from build123d import *

# Parameters (mm, degrees)
F1_DEPTH = 5
F2_W     = 240
F2_H     = 5
F3_DEPTH = 145
F5_DEPTH = 10
F6_DEPTH = 10


with BuildPart() as f1:
    # F0 (on Top) → F1 (new body)
    with BuildSketch(Plane.XY):
        Polygon((-126.897684, 95.248217), (-131.897684, 95.248217), (-131.897684, -154.751783), (118.102316, -154.751783), (118.102316, 95.248217), (113.102316, 95.248217), (113.102316, 81.383812), (-126.897684, 81.383812), align=None)
    extrude(amount=F1_DEPTH)

    # F2 (on face) → F3 (join)
    with BuildSketch(Plane.XY.offset(5)):
        Polygon((-126.897684, -149.751783), (-126.897684, 95.248217), (-131.897684, 95.248217), (-131.897684, -154.751783), (-126.897684, -154.751783), align=None)
        with Locations((-6.897684, -152.251783)):
            Rectangle(F2_W, F2_H)
        Polygon((113.102316, 95.248217), (113.102316, -149.751783), (113.102316, -154.751783), (118.102316, -154.751783), (118.102316, 95.248217), align=None)
    extrude(amount=F3_DEPTH)

    # F4 (on face) → F5 (join)
    with BuildSketch(Plane.XY.offset(150)):
        Polygon((-128.897684, -151.751783), (-6.897684, -151.751783), (-6.897684, -149.751783), (-126.897684, -149.751783), align=None)
        Polygon((-128.897684, 95.248217), (-128.897684, -151.751783), (-126.897684, -149.751783), (-126.897684, 95.248217), align=None)
    extrude(amount=F5_DEPTH)

    # F4 (on face) → F6 (join)
    with BuildSketch(Plane.XY.offset(150)):
        Polygon((118.102316, 95.248217), (116.102316, 95.248217), (116.102316, -152.751783), (118.102316, -154.751783), align=None)
        Polygon((118.102316, -154.751783), (116.102316, -152.751783), (-6.897684, -152.751783), (-6.897684, -154.751783), align=None)
    extrude(amount=F6_DEPTH)


solid = f1.part
Can you work these out from the model? Positions are in its coordinate system, mm. A direction names the side the tool comes from. Give positions to 0.01 mm unless a question says otherwise; leave off trailing zeros. Loops run counter-clockwise (first coordinate to the right, second up) from the corner with the lowest first, then second, coordinate; pieces in that order, holes last. Notation, with made-up numbers: M 4.5,58.5 L 55.5,58.5 A24 cw 55.5,83.5 Z; hole C -30.75,22 d10. An arc over 180 degrees is marked long. One line per item, written item: value. Start each with the question number.
1) Thinking about a two-plate mould opening in X: for faces 1 (the face through (-128.898, -27, 155)), 2 (the face through (113.102, -26, 74)), 3 (the face through (-9, -154.752, 79)), which applies, +X half, -X half, draft (parallel to the pull), parting line (faces both ways), or undercut?
2) If I drill on line 1 (X direction, y = 28.5, z = 110.5); line 2 (Y direction, x = 70, z = 109.5); line 3 (Z direction, x = -115, y = -28), over which ranges is the centre line in solid material (lowest first)? Write a range as [from, to].
3) I'm going to push flat-ended pins straight in: pin 1 (5.5 mm diameter, centred on x = -44.5, z = 1.5, fed in from +Y); pin 2 (11 mm diameter, centred on x = 49, z = 153.5, fed in from +Y); pin 3 (8 mm diameter, centred on y = -85.5, z = 154.5, fed in from -X); pin 4 (5 mm diameter, centred on x = 83, y = -89, fed in from -Z). Where does each tip first touch, or does it pass through?
4) If we section it at A-A, the plane z = 20: Write out the boundary of the cut face in (x, y), and give its area (3 significant figures).
5) If we section it at B-B, the plane y = -106.5: Write out the boundary of the cut face in (x, z), and give its area (3 significant figures).
6) If we section it at C-C, the plane x = -78.5: Write out the boundary of the cut face in (y, z), and give its area (3 significant figures).
7) On a 3-axis mill with a long thin cutter (end or side, diameter ignored), from which of +Z, -Z, +X, -X, +Y, -Y can I reach the whole of each face in a straight line? I mean faces 4 (the face through (118.102, -32, 79)), 5 (the face through (-69, -151.752, 155)), 6 (the face through (55, -152.752, 155)), 7 (the face through (-9, -33, 5)), 8 (the face through (-131.898, -28, 74)). Say none if no direction works.
Completed:
1. face 1: -X half
1. face 2: undercut
1. face 3: draft
2. line 1: x = [-131.9, -126.9], [113.1, 118.1]
2. line 2: y = [-154.75, -149.75]
2. line 3: z = [0, 5]
3. pin 1: stops at y = 81.38
3. pin 2: stops at y = -149.75
3. pin 3: stops at x = -128.9
3. pin 4: stops at z = 0
4. outline: M -131.9,-154.75 L 118.1,-154.75 L 118.1,95.25 L 113.1,95.25 L 113.1,-149.75 L -126.9,-149.75 L -126.9,95.25 L -131.9,95.25 Z
4. area: 3,700 mm^2
5. outline: M -131.9,0 L 118.1,0 L 118.1,160 L 116.1,160 L 116.1,150 L 113.1,150 L 113.1,5 L -126.9,5 L -126.9,160 L -128.9,160 L -128.9,150 L -131.9,150 Z
5. area: 2,740 mm^2
6. outline: M -154.75,0 L 81.38,0 L 81.38,5 L -149.75,5 L -149.75,160 L -151.75,160 L -151.75,150 L -154.75,150 Z
6. area: 1,930 mm^2
7. face 4: +Z, -Z, +X, +Y, -Y
7. face 5: +Z, -X, -Y
7. face 6: +Z, -X, +Y
7. face 7: +Z, +Y
7. face 8: +Z, -Z, -X, +Y, -Y
